The listing builds one solid part. Answer for the finished solid, in the listing's coordinates (mm). Coordinates: 2 decimals unless noted, no trailing zeros. Order: outer loops, then holes, each group sorted by start corner. A loop starts at its lowest first (then second) coordinate and runs counter-clockwise, first axis right, second up.
from build123d import *

# Parameters (mm, degrees)
SKETCH1_W               = 76.2
SKETCH1_H               = 76.2
BOSS_EXTRUDE1_DEPTH     = 19.05
F_1_4_CLEARANCE_HOLE1_D = 6.7564
F_2_CLEARANCE_HOLE1_D   = 2.4384
F_2_CLEARANCE_HOLE2_D   = 2.4384


with BuildPart() as part:
    # Sketch1 → Boss-Extrude1 (new body)
    with BuildSketch(Plane(origin=(0, 0, 0), x_dir=(1, 0, 0), z_dir=(0, 1, 0))):
        Rectangle(SKETCH1_W, SKETCH1_H)
    extrude(amount=BOSS_EXTRUDE1_DEPTH)

    # 1/4 Clearance Hole1 (through all)
    with Locations(Plane(origin=(0, 19.05, 0), x_dir=(1, 0, 0), z_dir=(0, 1, 0))):
        with Locations((0, 0)):
            Hole(F_1_4_CLEARANCE_HOLE1_D / 2)

    # #2 Clearance Hole1 (through all)
    with Locations(Plane(origin=(0, 19.05, 0), x_dir=(1, 0, 0), z_dir=(0, 1, 0))):
        with Locations((-12.7, 12.7), (0, 0)):
            Hole(F_2_CLEARANCE_HOLE1_D / 2)

    # #2 Clearance Hole2 (through all)
    with Locations(Plane(origin=(0, 19.05, 0), x_dir=(1, 0, 0), z_dir=(0, 1, 0))):
        with Locations((12.7, 12.7), (-12.7, -12.7), (12.7, -12.7)):
            Hole(F_2_CLEARANCE_HOLE2_D / 2)


solid = part.part
1) Section D-D (x = -2.5) is taken. Give the vertices of the cut face in (y, z), then the cut area to 3 significant figures.
2) Section A-A (z = -12.7) is taken. Give the vertices of the cut face in (x, y).
3) Consider L1, parallel to Z at x = 12.7, y = 9; L2, parallel to X at y = 15.5, z = -2.5. Determine where each line is inside the solid, lowest interval first.
4) Section B-B (x = -12.7) is taken. Give the vertices of the cut face in (y, z).
5) Section C-C (z = -2.5) is taken. Give the vertices of the cut face in (x, y).
6) Determine the mould class of faces 1 (the face through (-1, 9, -38.1)), 2 (the face through (2.681, 9.392, 2.056)), 3 (the face through (-38.1, 9, 1)), 4 (the face through (-13.263, 9.392, -11.618)) for opening direction Z: released by +Z, released by -Z, zero draft, split by the parting line, or undercut.
Filled sheet:
1. outline: (0, -38.1) - (19.05, -38.1) - (19.05, -2.27) - (0, -2.27) - close; (0, 2.27) - (19.05, 2.27) - (19.05, 38.1) - (0, 38.1) - close
1. area: 1,370 mm2
2. outline: (-38.1, 0) - (-13.92, 0) - (-13.92, 19.05) - (-38.1, 19.05) - close; (-11.48, 0) - (11.48, 0) - (11.48, 19.05) - (-11.48, 19.05) - close; (13.92, 0) - (38.1, 0) - (38.1, 19.05) - (13.92, 19.05) - close
3. L1: z = -38.1 to -13.92, -11.48 to 11.48, 13.92 to 38.1
3. L2: x = -38.1 to -2.27, 2.27 to 38.1
4. outline: (0, -38.1) - (19.05, -38.1) - (19.05, -13.92) - (0, -13.92) - close; (0, -11.48) - (19.05, -11.48) - (19.05, 11.48) - (0, 11.48) - close; (0, 13.92) - (19.05, 13.92) - (19.05, 38.1) - (0, 38.1) - close
5. outline: (-38.1, 0) - (-2.27, 0) - (-2.27, 19.05) - (-38.1, 19.05) - close; (2.27, 0) - (38.1, 0) - (38.1, 19.05) - (2.27, 19.05) - close
6. face 1: released by -Z
6. face 2: undercut
6. face 3: zero draft
6. face 4: undercut
